For this review, take the finished solid that the model builds, in its own axes (mm). Coordinates: 2 decimals unless noted, no trailing zeros. Loops run counter-clockwise (first coordinate to the right, second up) from the corner with the lowest first, then second, coordinate; pieces in that order, holes last. Notation, with made-up numbers: (-24.5, 22) -> (15.5, 22) arc R13 ccw to (15.5, 27) -> close; hole circle Ø5 at (56, 89.5). An arc over 180 degrees is marked (long way). One line per item, written item: value.
from build123d import *

# Parameters (mm, degrees)
F0_W     = 347.3
F0_H     = 51.58
F0_R     = 4.7625
F0_R_2   = 12.5
F1_DEPTH = 6.35
F3_D     = 6.6
F5_D     = 2.5


with BuildPart() as f1:
    # F0 (on Top) → F1 (new body)
    with BuildSketch(Plane.XY):
        Rectangle(F0_W, F0_H)
        with Locations((-123.65, 0)):
            Circle(F0_R, mode=Mode.SUBTRACT)
        Circle(F0_R_2, mode=Mode.SUBTRACT)
        with Locations((123.65, 0)):
            Circle(F0_R, mode=Mode.SUBTRACT)
    extrude(amount=F1_DEPTH)

    # F3 (through all)
    with Locations(Plane(origin=(0, 0, 0), x_dir=(1, 0, 0), z_dir=(0, 0, -1))):
        with Locations((-160.553125, 12.895), (-160.553125, -12.895), (160.553125, 12.895), (160.553125, -12.895)):
            Hole(F3_D / 2)

    # F5 (through all)
    with Locations(Plane.XY.offset(6.35)):
        with Locations((-123.65, 8), (-115.65, 0), (-123.65, -8), (-131.65, 0), (123.65, 8), (131.65, 0), (123.65, -8), (115.65, 0)):
            Hole(F5_D / 2)


solid = f1.part
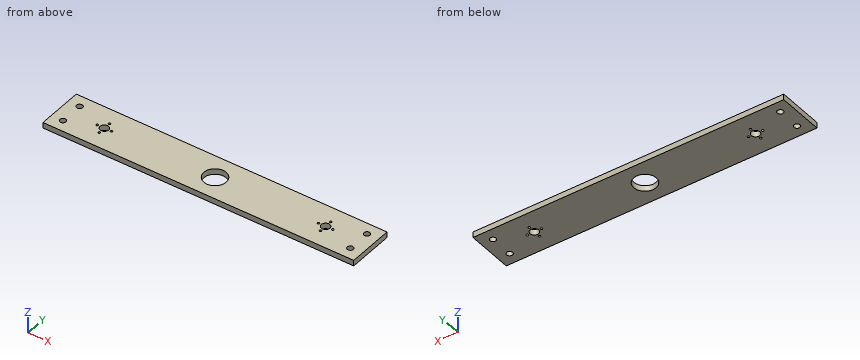
1. Insertion check: pin 1 Ø2 at (x, y) = (-132.5, -10.5) entering from -Z. The pin has a flat end and moves straight along its axis. Give the tip position at first contact, or say it passes through.
Return value:
pin 1: stops at z = 0
2. Take a section at B-B, the plane z = 4.75. Give the number of separate pieces and of enclosed holes in the cut face, and give its area (3 significant figures).
Return value:
separate pieces: 1
enclosed holes: 15
area: 17,100 mm2
3. Take a section at A-A, the plane x = 0. Give the boundary of the cut face in (y, z), and give its area (3 significant figures).
Return value:
outline: (-25.79, 0) -> (-12.5, 0) -> (-12.5, 6.35) -> (-25.79, 6.35) -> close; (12.5, 0) -> (25.79, 0) -> (25.79, 6.35) -> (12.5, 6.35) -> close
area: 169 mm2
4. To check wall thickness, follow probe 1 along Y at (x, z) = (-123.65, 3.5); probe 2 along Y at (x, z) = (0, 1.75); probe 3 along X at (y, z) = (10, 0.75). State the ranges of each line that lie inside material, in increasing order. Write a range as from..to.
Return value:
probe 1: y = -25.79..-9.25, -6.75..-4.76, 4.76..6.75, 9.25..25.79
probe 2: y = -25.79..-12.5, 12.5..25.79
probe 3: x = -173.65..-162.14, -158.97..-7.5, 7.5..158.97, 162.14..173.65
